Part print with two shaded views. Sizes in mm from the minimum x, y, z corner. Round coordinates to 2 decimals unless told otherwise and drop trailing zeros. Order: outer loops, then holes, each group sorted by start corner. A loop starts at its lowest first (then second) coordinate and runs counter-clockwise, first axis right, second up. Notation, with made-up numbers: (-40, 80.25) -> (-2, 80.25) arc R24 ccw to (-2, 99.25) -> close; hole circle Ø1 at (42.25, -12.5). An arc over 180 degrees is marked (long way). Use a Markdown table: item, result. Add a question column.
Item 1: Probe L1, parallel to X at y = 30.5, z = 14.75; L2, parallel to X at y = 86.5, z = 16.5; L3, parallel to X at y = 22, z = 18. List the from-to ranges inside material, lowest first.
Item 2: Pin check, flat tips, straight feed: pin 1 (1.5 mm diameter, centred on x = 126.5, z = 10, fed in from -Y); pin 2 (16.5 mm diameter, centred on x = 275.5, y = 33, fed in from +Z); pin 3 (12 mm diameter, centred on x = 126, z = 4.5, fed in from -Y). Stop position of each tip, or through.
Item 3: Slice it at D-D, the plane y = 85. Give the cut face in (x, z).
Item 4: Slice it at A-A, the plane y = 43. Give the cut face in (x, z).
Item 5: Slice it at C-C, the plane x = 39. Give the cut face in (y, z), plus the area to 3 significant figures.
Item 6: Slice it at B-B, the plane z = 15. Give the cut face in (x, y), plus the area to 3 significant figures.
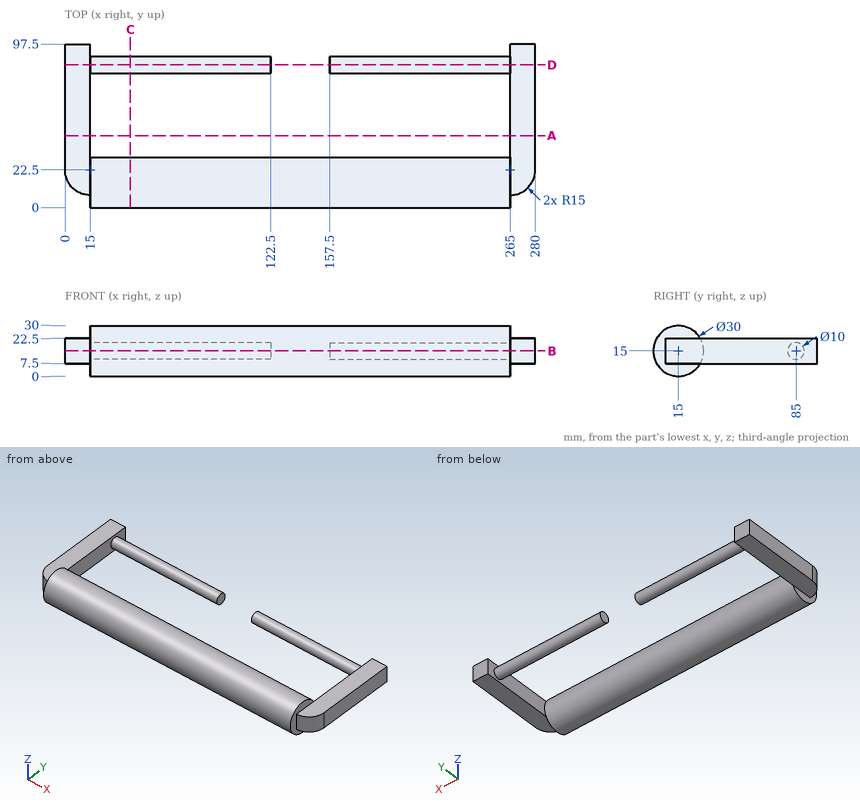
Check sheet entries:
| question | item | result |
|---|---|---|
| 1 | L1 | 0 to 15, 265 to 280 |
| 1 | L2 | 0 to 122.5, 157.5 to 280 |
| 1 | L3 | 0.01 to 279.99 |
| 2 | pin 1 | y = 0.61 |
| 2 | pin 2 | z = 22.5 |
| 2 | pin 3 | y = 0.69 |
| 3 | outline | (0, 7.5) -> (15, 7.5) -> (15, 10) -> (122.5, 10) -> (122.5, 20) -> (15, 20) -> (15, 22.5) -> (0, 22.5) -> close; (157.5, 10) -> (265, 10) -> (265, 7.5) -> (280, 7.5) -> (280, 22.5) -> (265, 22.5) -> (265, 20) -> (157.5, 20) -> close |
| 4 | outline | (0, 7.5) -> (15, 7.5) -> (15, 22.5) -> (0, 22.5) -> close; (265, 7.5) -> (280, 7.5) -> (280, 22.5) -> (265, 22.5) -> close |
| 5 | outline | circle Ø30 at (15, 15); circle Ø10 at (85, 15) |
| 5 | area | 785 mm2 |
| 6 | outline | (0, 22.5) arc R15 ccw to (15, 7.5) -> (15, 0) -> (265, 0) -> (265, 7.5) arc R15 ccw to (280, 22.5) -> (280, 97.5) -> (265, 97.5) -> (265, 90) -> (157.5, 90) -> (157.5, 80) -> (265, 80) -> (265, 30) -> (15, 30) -> (15, 80) -> (122.5, 80) -> (122.5, 90) -> (15, 90) -> (15, 97.5) -> (0, 97.5) -> close |
| 6 | area | 12,300 mm2 |
